Part model, mm, in its own coordinate system. A direction names the side the tool comes from. Coordinates: 2 decimals unless noted, no trailing zeros. Order: outer loops, then holes, each group sorted by start corner. A loop starts at its lowest first (then second) coordinate and runs counter-clockwise, first axis right, second up.
1) Cut at B-B (z = 0). Give the number of separate pieces and of enclosed holes in the cut face, and give its area (3 significant figures).
2) Cut at C-C (y = 38.5). List the corners of the cut face in (x, z) (3 decimals).
3) Cut at D-D (y = 47). List the corners of the cut face in (x, z).
4) Pin check, flat tips, straight feed: pin 1 Ø2 at (x, y) = (-2, 10) entering from -Z; pin 2 Ø1.4 at (x, y) = (9, 46) entering from +Z; pin 3 Ø2 at (x, z) = (-2, -8.5) entering from -Y. Stop position of each tip, or through.
5) Tool access for faces 1 (the flat face through (1, 27, -15.3)), 2 (the flat face through (-6.805, 20.28, 8.363)), 3 (the flat face through (7, 20, 3.8)), 4 (the flat face through (-8, 46, -6.8)): list every direction of +Z, -Z, +X, -X, +Y, -Y with a clear straight run to the whole face (end or side of a thin tool).
6) Mould opens along Y. For faces 5 (the flat face through (-2, 44.1, -15)), 6 (the flat face through (0, 52, -14)), 7 (the flat face through (8, 12, -16.8)) say: +Y half, -Y half, draft (parallel to the pull), parting line (faces both ways), or undercut.
7) Cut at A-A (x = -4.5). List the corners of the cut face in (y, z), and give its area (3 significant figures).
8) Wall check: L1, parallel to X at y = 39, z = 0 (3 decimals); L2, parallel to X at y = 14, z = 0; L3, parallel to Y at x = -10, z = -6. Give the ranges that are in metal, low to high.
```python
from build123d import *

# Parameters (mm, degrees)
EXTRUDE_1_DEPTH      = 40
SKETCH_2_R           = 1.5
CUT_EXTRUDE_1_DEPTH  = 47.523972315
CUT_EXTRUDE_2_DEPTH  = 47.523972315
EXTRUDE_2_DEPTH      = 12
SKETCH_5_W           = 12
SKETCH_5_H           = 8.5
CUT_EXTRUDE_3_DEPTH  = 47.523972315
CUT_EXTRUDE_4_DEPTH  = 12
SKETCH_7_W           = 2.5
SKETCH_7_H           = 5
EXTRUDE_3_DEPTH      = 5.3
SKETCH_8_W           = 2.5
SKETCH_8_H           = 5
EXTRUDE_4_DEPTH      = 5.2
SKETCH_10_W          = 16
SKETCH_10_H          = 8.5
CUT_EXTRUDE_5_DEPTH  = 47.523972315
SKETCH_11_W          = 7.5
SKETCH_11_H          = 4.1
CUT_EXTRUDE_6_DEPTH  = 11
SKETCH_15_W          = 7.5
SKETCH_15_H          = 5
CUT_EXTRUDE_10_DEPTH = 10
SKETCH_12_W          = 7.5
SKETCH_12_H          = 1.5
CUT_EXTRUDE_7_DEPTH  = 28
CUT_EXTRUDE_START    = -20
CUT_EXTRUDE_8_DEPTH  = 5
FILLET_2_R           = 2
SKETCH_16_R          = 3.025
CUT_EXTRUDE_11_DEPTH = 2.2
SKETCH_17_W          = 1.5
SKETCH_17_H          = 4
CUT_EXTRUDE_12_DEPTH = 40.855739863
FILLET_3_R           = 1


with BuildPart() as part:
    # 草图1 → 凸台-拉伸1 (new body)
    with BuildSketch(Plane(origin=(0, 0, 0), x_dir=(1, 0, 0), z_dir=(0, 1, 0))):
        Polygon((11.908535316, 16.8), (-11.908535316, 16.8), (-16.8, 11.908535316), (-16.8, -11.908535316), (-11.908535316, -16.8), (11.908535316, -16.8), (16.8, -11.908535316), (16.8, 11.908535316), align=None)
    extrude(amount=EXTRUDE_1_DEPTH)

    # 草图2 → 切除-拉伸1 (cut, through all)
    with BuildSketch(Plane(origin=(0, 40, 0), x_dir=(1, 0, 0), z_dir=(0, 1, 0))):
        with Locations(Location((12, 0, 0), (0, 0, 270))):
            Circle(SKETCH_2_R)
        with Locations(Location((-12, 0, 0), (0, 0, 90))):
            Circle(SKETCH_2_R)
    extrude(amount=-CUT_EXTRUDE_1_DEPTH, mode=Mode.SUBTRACT)

    # 草图3 → 切除-拉伸2 (cut, through all)
    with BuildSketch(Plane(origin=(0, 40, 0), x_dir=(1, 0, 0), z_dir=(0, 1, 0))):
        Polygon((-6, -3.8), (6, -3.8), (7.586942826, -12.8), (13, -12.8), (13, -16.8), (-13, -16.8), (-13, -12.8), (-7.586942826, -12.8), align=None)
    extrude(amount=-CUT_EXTRUDE_2_DEPTH, mode=Mode.SUBTRACT)

    # 草图4 → 凸台-拉伸2 (add)
    with BuildSketch(Plane(origin=(0, 40, 0), x_dir=(1, 0, 0), z_dir=(0, 1, 0))):
        Polygon((-10, 16.8), (-10, 6.8), (-6, 6.8), (-6, 13.3), (7.2, 13.3), (7.2, 6.8), (10, 6.8), (10, 16.8), align=None)
    extrude(amount=EXTRUDE_2_DEPTH)

    # 草图5 → 切除-拉伸3 (cut, through all)
    with BuildSketch(Plane(origin=(0, 40, 0), x_dir=(1, 0, 0), z_dir=(0, 1, 0))):
        with Locations((0, 0.45)):
            Rectangle(SKETCH_5_W, SKETCH_5_H)
    extrude(amount=-CUT_EXTRUDE_3_DEPTH, mode=Mode.SUBTRACT)

    # 草图6 → 切除-拉伸4 (cut)
    with BuildSketch(Plane.XZ):
        Polygon((-6, -6.8), (-6, -13.3), (-6, -16.8), (7.2, -16.8), (7.2, -13.3), (7.2, -6.8), align=None)
    extrude(amount=-CUT_EXTRUDE_4_DEPTH, mode=Mode.SUBTRACT)

    # 草图7 → 凸台-拉伸3 (add)
    with BuildSketch(Plane(origin=(0, 40, 0), x_dir=(1, 0, 0), z_dir=(0, 1, 0))):
        with Locations((2.75, 10.8)):
            Rectangle(SKETCH_7_W, SKETCH_7_H)
        with Locations((-2.25, 10.8)):
            Rectangle(SKETCH_7_W, SKETCH_7_H)
    extrude(amount=EXTRUDE_3_DEPTH)

    # 草图8 → 凸台-拉伸4 (add)
    with BuildSketch(Plane.XZ.offset(-12)):
        with Locations((-2.25, -9.3)):
            Rectangle(SKETCH_8_W, SKETCH_8_H)
        with Locations((2.75, -9.3)):
            Rectangle(SKETCH_8_W, SKETCH_8_H)
    extrude(amount=EXTRUDE_4_DEPTH)

    # 草图10 → 切除-拉伸5 (cut, through all)
    with BuildSketch(Plane(origin=(0, 40, 0), x_dir=(1, 0, 0), z_dir=(0, 1, 0))):
        with Locations((0, 0.45)):
            Rectangle(SKETCH_10_W, SKETCH_10_H)
    extrude(amount=-CUT_EXTRUDE_5_DEPTH, mode=Mode.SUBTRACT)

    # 草图11 → 切除-拉伸6 (cut)
    with BuildSketch(Plane.XY.offset(-13.3)):
        with Locations((-2.25, 42.05)):
            Rectangle(SKETCH_11_W, SKETCH_11_H)
    extrude(amount=-CUT_EXTRUDE_6_DEPTH, mode=Mode.SUBTRACT)

    # 草图15 → 切除-拉伸10 (cut)
    with BuildSketch(Plane(origin=(0, 0, -16.8), x_dir=(-1, 0, 0), z_dir=(0, 0, -1))):
        with Locations((2.25, 14.5)):
            Rectangle(SKETCH_15_W, SKETCH_15_H)
    extrude(amount=-CUT_EXTRUDE_10_DEPTH, mode=Mode.SUBTRACT)

    # 草图12 → 切除-拉伸7 (cut)
    with BuildSketch(Plane(origin=(0, 40, 0), x_dir=(1, 0, 0), z_dir=(0, 1, 0))):
        with Locations((-2.25, 16.05)):
            Rectangle(SKETCH_12_W, SKETCH_12_H)
    extrude(amount=-CUT_EXTRUDE_7_DEPTH, mode=Mode.SUBTRACT)

    # 草图13 → 切除-拉伸8 (cut)
    with BuildSketch(Plane.XZ.offset(CUT_EXTRUDE_START)):
        Polygon((11.908535316, -16.8), (1.5, -16.8), (1.5, -15.3), (11.287214973, -15.3), (15.3, -11.287214973), (15.3, -5.908535316), (16.8, -5.908535316), (16.8, -11.908535316), align=None)
    extrude(amount=-CUT_EXTRUDE_8_DEPTH, mode=Mode.SUBTRACT)

    # 圆角2
    fillet_2_edges = [part.edges().sort_by_distance(p)[0] for p in [
        (-2.25, 17, -15.3),
    ]]
    fillet(fillet_2_edges, radius=FILLET_2_R)

    # 草图16 → 切除-拉伸11 (cut)
    with BuildSketch(Plane(origin=(0, 40, 0), x_dir=(1, 0, 0), z_dir=(0, 1, 0))):
        with Locations(Location((12, 0, 0), (0, 0, 270))):
            Circle(SKETCH_16_R)
        with Locations(Location((-12, 0, 0), (0, 0, 270))):
            Circle(SKETCH_16_R)
    cut_extrude_11 = extrude(amount=-CUT_EXTRUDE_11_DEPTH, mode=Mode.SUBTRACT)

    # 镜向1: 切除-拉伸11 across plane
    add(cut_extrude_11.mirror(Plane.ZX.offset(20)), mode=Mode.SUBTRACT)

    # 草图17 → 切除-拉伸12 (cut, through all)
    with BuildSketch(Plane(origin=(0, 20, 0), x_dir=(1, 0, 0), z_dir=(0, 1, 0))):
        with Locations((16.05, 7.908535316)):
            Rectangle(SKETCH_17_W, SKETCH_17_H)
    extrude(amount=-CUT_EXTRUDE_12_DEPTH, mode=Mode.SUBTRACT)

    # 圆角3
    fillet_3_edges = [part.edges().sort_by_distance(p)[0] for p in [
        (1.5, 25, -16.05),
        (1.5, 20, -16.05),
        (16.05, 20, -9.908535316),
    ]]
    fillet(fillet_3_edges, radius=FILLET_3_R)


solid = part.part
```
Geometry check:
1. separate pieces: 4
1. enclosed holes: 0
1. area: 437 mm2
2. outline: (-16.8, -11.909) - (-11.909, -16.8) - (-6, -16.8) - (-6, -15.3) - (1.5, -15.3) - (1.5, -16.8) - (11.909, -16.8) - (16.8, -11.909) - (16.8, 11.909) - (13, 15.709) - (13, 12.8) - (7.587, 12.8) - (6, 3.8) - (8, 3.8) - (8, -4.7) - (-8, -4.7) - (-8, 3.8) - (-6, 3.8) - (-7.587, 12.8) - (-13, 12.8) - (-13, 15.709) - (-16.8, 11.909) - close; hole circle Ø6.05 at (-12, 0); hole circle Ø6.05 at (12, 0)
3. outline: (-10, -16.8) - (10, -16.8) - (10, -6.8) - (7.2, -6.8) - (7.2, -13.3) - (-6, -13.3) - (-6, -6.8) - (-10, -6.8) - close
4. pin 1: stops at z = -11.8
4. pin 2: stops at z = -6.8
4. pin 3: stops at y = 6.8
5. face 1: -Z
5. face 2: +Z, +Y, -Y
5. face 3: +Y, -Y
5. face 4: +Z, +X, -X, +Y
6. face 5: undercut
6. face 6: +Y half
6. face 7: draft
7. outline: (0, -6.8) - (17, -6.8) - (17, -13.3) arc R2 ccw to (19, -15.3) - (40, -15.3) - (40, -4.7) - (0, -4.7) - close; (44.1, -16.8) - (52, -16.8) - (52, -13.3) - (44.1, -13.3) - close
7. area: 306 mm2
8. L1: x = -16.8 to -15.025, -8.975 to -8, 8 to 8.975, 15.025 to 16.8
8. L2: x = -16.8 to -13.5, -10.5 to -8, 8 to 10.5, 13.5 to 16.8
8. L3: y = 0 to 40
